Design review of the part built by this model. Coordinates are the model's own, in mm. Give positions to 0.01 mm unless a question says otherwise; leave off trailing zeros. Loops run counter-clockwise (first coordinate to the right, second up) from the corner with the lowest first, then second, coordinate; pieces in that order, holes last. Notation, with made-up numbers: (69.25, -24) - (85.25, -24) arc R21 cw to (85.25, 0) - close; hole circle Ø1 at (-6, 89). An arc over 180 degrees is marked (long way). Put each result on its own line as item: value. Start each with the question number.
Autodesk Inventor part; units mm, degrees
ref_plane "YZ Plane" through (0, 0, 0) normal (1, 0, 0) x (0, 1, 0)
ref_plane "XZ Plane" through (0, 0, 0) normal (0, 1, 0) x (-1, 0, 0)
ref_plane "XY Plane" through (0, 0, 0) normal (0, 0, 1) x (1, 0, 0)
sketch "Sketch1" plane through (0, 0, 0) normal (0, 1, 0) x (-1, 0, 0)
  line L0 (25, 25) -> (-25, 25)
  line L1 (-25, 25) -> (-25, -25)
  line L2 (-25, -25) -> (25, -25)
  line L3 (25, -25) -> (25, 25)
  line L4 (25, 25) -> (-25, -25) construction
  line L5 (-25, 25) -> (25, -25) construction
  line L6 (6, 6) -> (-6, 6)
  line L7 (-6, 6) -> (-6, -6)
  line L8 (-6, -6) -> (6, -6)
  line L9 (6, -6) -> (6, 6)
  line L10 (6, 6) -> (-6, -6) construction
  line L11 (-6, 6) -> (6, -6) construction
  line L12 (20, 20) -> (-20, 20) construction
  line L13 (-20, 20) -> (-20, -20) construction
  line L14 (-20, -20) -> (20, -20) construction
  line L15 (20, -20) -> (20, 20) construction
  line L16 (20, 20) -> (-20, -20) construction
  line L17 (-20, 20) -> (20, -20) construction
  circle A0 centre (20, 20) radius 2.625
  circle A1 centre (20, -20) radius 2.625
  circle A2 centre (-20, -20) radius 2.625
  circle A3 centre (-20, 20) radius 2.625
  point P0 (0, 0)
  dimension "d0" = 50
  dimension "d1" = 50
  dimension "d2" = 12
  dimension "d3" = 12
  dimension "d4" = 40
  dimension "d5" = 40
  dimension "d6" = 5.25
  dimension "d7" = 5.25
  dimension "d8" = 5.25
  dimension "d9" = 5.25
extrude "Extrusion1" add sketch "Sketch1" along normal blind 2
fillet "Fillet1" radius 3.5 4 edges at (-6, 1, 6) (-6, 1, -6) (6, 1, -6) (6, 1, 6)
properties part number "arena_middle"
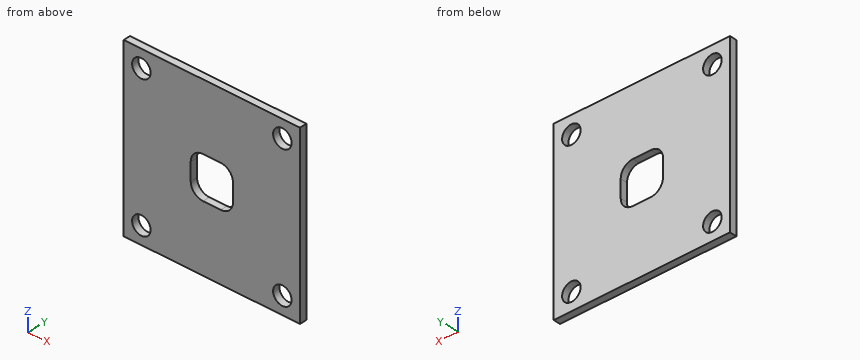
Item 1: Consider section C-C (x = -20). State the section outline as (y, z) points (3 decimals).
Item 2: Consider section B-B (y = 1.5). State the section outline as (x, z) points (3 decimals), plus the area to 3 significant figures.
Item 3: Consider section A-A (z = 20). State the section outline as (x, y) points (3 decimals), plus the area to 3 significant figures.
Item 4: For L1, parallel to Z at x = -20, y = 0.5 (3 decimals); L2, parallel to Z at x = 22, y = 1.85; L3, parallel to X at y = 0.65, z = -2.5, list the stretches that pass through material, from the lowest coordinate up. Write a range as from..to.
Geometry says:
1. outline: (0, -25) - (2, -25) - (2, -22.625) - (0, -22.625) - close; (0, -17.375) - (2, -17.375) - (2, 17.375) - (0, 17.375) - close; (0, 22.625) - (2, 22.625) - (2, 25) - (0, 25) - close
2. outline: (-25, -25) - (25, -25) - (25, 25) - (-25, 25) - close; hole circle Ø5.25 at (-20, -20); hole circle Ø5.25 at (-20, 20); hole (-6, -2.5) arc R3.5 ccw to (-2.5, -6) - (2.5, -6) arc R3.5 ccw to (6, -2.5) - (6, 2.5) arc R3.5 ccw to (2.5, 6) - (-2.5, 6) arc R3.5 ccw to (-6, 2.5) - close; hole circle Ø5.25 at (20, -20); hole circle Ø5.25 at (20, 20)
2. area: 2,280 mm2
3. outline: (-25, 0) - (-22.625, 0) - (-22.625, 2) - (-25, 2) - close; (-17.375, 0) - (17.375, 0) - (17.375, 2) - (-17.375, 2) - close; (22.625, 0) - (25, 0) - (25, 2) - (22.625, 2) - close
3. area: 79.0 mm2
4. L1: z = -25..-22.625, -17.375..17.375, 22.625..25
4. L2: z = -25..-21.7, -18.3..18.3, 21.7..25
4. L3: x = -25..-6, 6..25
